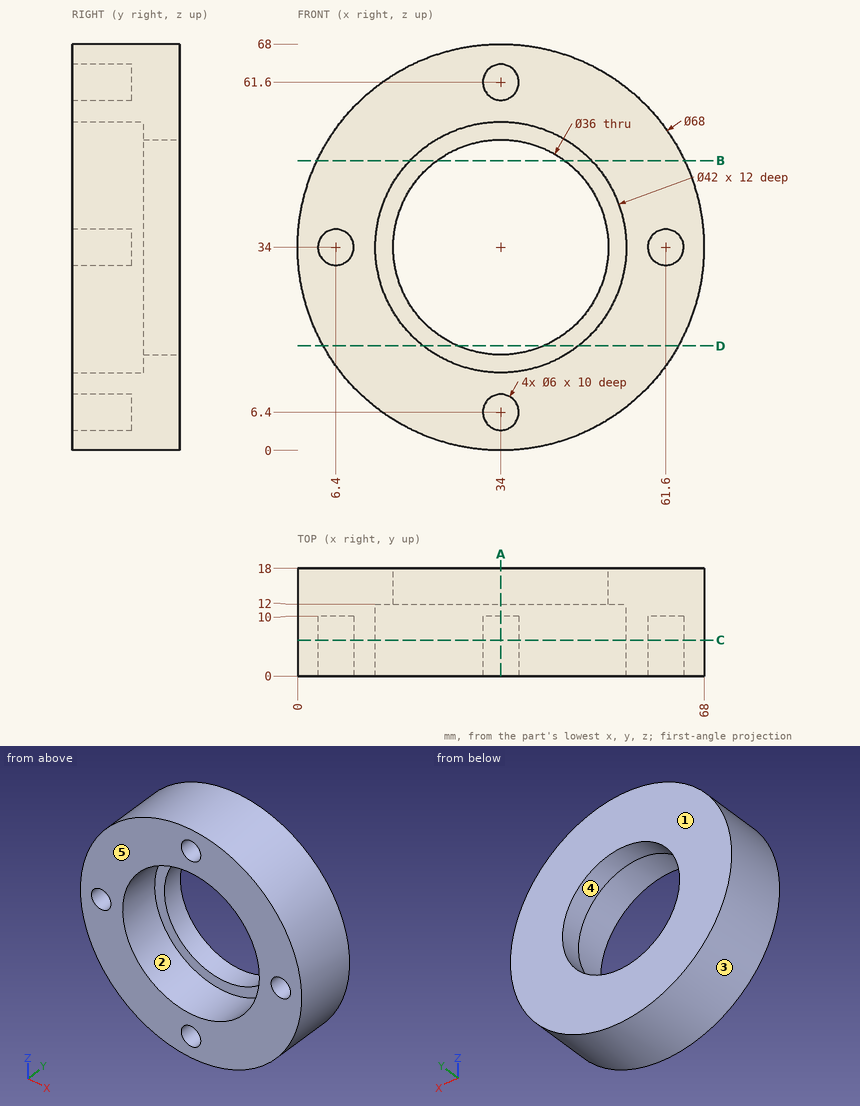
Drawing for the job (mm, zero at the part's lowest x, y, z). A direction names the side the tool comes from. Round coordinates to 2 decimals unless told otherwise and drop trailing zeros. Loops run counter-clockwise (first coordinate to the right, second up) from the corner with the lowest first, then second, coordinate; pieces in that order, holes last.
1. Drop flat-ended pins along their axis: P1, Ø21, axis at x = 39, z = 33.5, coming from the -Y side (1 decimal); P2, Ø2, axis at x = 12, y = 12.5, coming from the -Z side; P3, Ø10, axis at y = 5.5, z = 29, coming from the -X side; P4, Ø3, axis at x = 61.5, z = 33, coming from the -Y side. Give the stop position or say it passes through.
Check values:
P1: passes through
P2: stops at z = 7.26
P3: stops at x = 0
P4: stops at y = 10
2. Band-saw the part on D-D, the plane z = 17.5. List the corners of the cut face in (x, y).
Check values:
outline: (4.27, 0) - (21.01, 0) - (21.01, 12) - (26.81, 12) - (26.81, 18) - (4.27, 18) - close; (41.19, 12) - (46.99, 12) - (46.99, 0) - (63.73, 0) - (63.73, 18) - (41.19, 18) - close
3. Tool access for the marked faces 1 and 2: list every direction of +Z, -Z, +X, -X, +Y, -Y with a clear straight run to the whole face (end or side of a thin tool).
Check values:
face 1: +Z, -Z, +X, -X, +Y
face 2: -Y
4. Mould opens along Z. For the marked faces 3, 4 and 5 say: +Z half, -Z half, draft (parallel to the pull), parting line (faces both ways), or undercut.
Check values:
face 3: parting line
face 4: undercut
face 5: draft
5. Wall check: probe 1 along X at (y, z) = (4.5, 34); probe 2 along X at (y, z) = (16.25, 34.5); probe 3 along Z at (x, y) = (46.5, 8.25). Give the ranges that are in metal, low to high.
Check values:
probe 1: x = 0 to 3.4, 9.4 to 13, 55 to 58.6, 64.6 to 68
probe 2: x = 0 to 16.01, 51.99 to 68
probe 3: z = 2.38 to 17.13, 50.87 to 65.62
6. Band-saw the part on B-B, the plane z = 48.5. List the corners of the cut face in (x, y).
Check values:
outline: (3.25, 0) - (18.81, 0) - (18.81, 12) - (23.33, 12) - (23.33, 18) - (3.25, 18) - close; (44.67, 12) - (49.19, 12) - (49.19, 0) - (64.75, 0) - (64.75, 18) - (44.67, 18) - close
7. Band-saw the part on A-A, the plane x = 34. List the corners of the cut face in (y, z), and give its area (3 significant figures).
Check values:
outline: (0, 0) - (18, 0) - (18, 16) - (12, 16) - (12, 13) - (0, 13) - (0, 9.4) - (10, 9.4) - (10, 3.4) - (0, 3.4) - close; (0, 55) - (12, 55) - (12, 52) - (18, 52) - (18, 68) - (0, 68) - (0, 64.6) - (10, 64.6) - (10, 58.6) - (0, 58.6) - close
area: 384 mm2
8. Band-saw the part on C-C, the plane y = 6. List the corners of the cut face in (x, z).
Check values:
outline: circle Ø68 at (34, 34); hole circle Ø6 at (6.4, 34); hole circle Ø42 at (34, 34); hole circle Ø6 at (34, 6.4); hole circle Ø6 at (34, 61.6); hole circle Ø6 at (61.6, 34)
